Input: part model. Units: mm. Frame: model coordinates. A direction names the side the tool comes from. Coordinates: 2 decimals unless noted, no trailing zeros. Order: outer loops, then holes, each group sorted by start corner. A loop starts at its lowest first (then second) coordinate and runs counter-clockwise, first axis right, second up. Notation, with made-up numbers: M 17,55 L 70,55 A21 ccw 70,79 Z; hole C -36,77.25 d6. An arc over 180 degrees is marked long. Answer in a Markdown table with one row per item.
from build123d import *

# Parameters (mm, degrees)
SKETCH_1_W          = 830
SKETCH_1_H          = 82.91
EXTRUDE_2_DEPTH     = 20
SKETCH_4_W          = 830
SKETCH_4_H          = 10
CUT_EXTRUDE_3_DEPTH = 70
SKETCH_5_W          = 830
SKETCH_5_H          = 15
EXTRUDE_3_DEPTH     = 3.28
SKETCH_6_W          = 3.54
SKETCH_6_H          = 69.4
EXTRUDE_5_DEPTH     = 200.2
SKETCH_8_W          = 20
SKETCH_8_H          = 10.39973114
CUT_EXTRUDE_5_DEPTH = 1000.2
SKETCH_9_W          = 8.730890719
SKETCH_9_H          = 180.752173936
EXTRUDE_6_DEPTH     = 3.62
SKETCH_10_W         = 3.09
SKETCH_10_H         = 69.4
EXTRUDE_7_DEPTH     = 820
SKETCH_13_W         = 830
SKETCH_13_H         = 20
EXTRUDE_18_DEPTH    = 3.85


with BuildPart() as part:
    # 草图1 → 凸台-拉伸2 (new body)
    with BuildSketch(Plane.XY):
        with Locations((337.654216889, 6.096927721)):
            Rectangle(SKETCH_1_W, SKETCH_1_H)
    extrude(amount=EXTRUDE_2_DEPTH)

    # 草图4 → 切除-拉伸3 (cut)
    with BuildSketch(Plane(origin=(0, 47.551927721, 0), x_dir=(1, 0, 0), z_dir=(0, 1, 0))):
        with Locations((337.654216889, -15)):
            Rectangle(SKETCH_4_W, SKETCH_4_H)
    extrude(amount=-CUT_EXTRUDE_3_DEPTH, mode=Mode.SUBTRACT)

    # 草图5 → 凸台-拉伸3 (add)
    with BuildSketch(Plane(origin=(0, 47.551927721, 0), x_dir=(1, 0, 0), z_dir=(0, 1, 0))):
        with Locations((337.654216889, -7.5)):
            Rectangle(SKETCH_5_W, SKETCH_5_H)
    extrude(amount=EXTRUDE_3_DEPTH)

    # 草图6 → 凸台-拉伸5 (add)
    with BuildSketch(Plane(origin=(752.654216889, 50.831927721, 0), x_dir=(-1, 0, 0), z_dir=(0, 0, -1))):
        with Locations((1.77, -37.215224989)):
            Rectangle(SKETCH_6_W, SKETCH_6_H)
    extrude(amount=-EXTRUDE_5_DEPTH)

    # 草图8 → 切除-拉伸5 (cut)
    with BuildSketch(Plane.ZY.offset(77.345783111)):
        with Locations((10, -30.158206709)):
            Rectangle(SKETCH_8_W, SKETCH_8_H)
    extrude(amount=-CUT_EXTRUDE_5_DEPTH, mode=Mode.SUBTRACT)

    # 草图9 → 凸台-拉伸6 (add)
    with BuildSketch(Plane.XZ.offset(21.083297268)):
        with Locations((748.455599967, 110.153891103)):
            Rectangle(SKETCH_9_W, SKETCH_9_H)
    extrude(amount=EXTRUDE_6_DEPTH)

    # 草图10 → 凸台-拉伸7 (add)
    with BuildSketch(Plane.ZY.offset(-749.114216889)):
        with Locations((99.616509489, 13.616702732)):
            Rectangle(SKETCH_10_W, SKETCH_10_H)
    extrude(amount=EXTRUDE_7_DEPTH)

    # 草图13 → 凸台-拉伸18 (add)
    with BuildSketch(Plane(origin=(0, 48.316702732, 0), x_dir=(1, 0, 0), z_dir=(0, 1, 0))):
        with Locations((337.654216889, -108.539027645)):
            Rectangle(SKETCH_13_W, SKETCH_13_H)
    extrude(amount=EXTRUDE_18_DEPTH)


solid = part.part
1) Reachability of faces 4 (the face through (-77.346, 12, 3)), 5 (the face through (749.114, 13, 150)), 6 (the face through (332, 50.832, 7)) from +Z, -Z, +X, -X, +Y, -Y: full face, straight path, thin tool, end or side. Return the list, or none.
Resolved:
| item | result |
|---|---|
| face 4 | +Z, -Z, -X, +Y, -Y |
| face 5 | +Z, -X |
| face 6 | -Z, +X, -X, +Y |
2) Material intervals for probe 1 along Z at (x, y) = (318, 12.5); probe 2 along X at (y, z) = (29, 46), sorted ascending.
Resolved:
| item | result |
|---|---|
| probe 1 | z = 0 to 10, 98.07 to 101.16 |
| probe 2 | x = 749.11 to 752.65 |
3) Cut plane A-A, the plane x = 361. Output: boundary loops of the cut face in (y, z).
Resolved:
| item | result |
|---|---|
| outline | M -24.96,0 L 50.83,0 L 50.83,15 L 47.55,15 L 47.55,10 L -22.45,10 L -22.45,20 L -24.96,20 Z; M -21.08,98.07 L 48.32,98.07 L 48.32,98.54 L 52.17,98.54 L 52.17,118.54 L 48.32,118.54 L 48.32,101.16 L -21.08,101.16 Z |
4) Cut plane C-C, the plane z = 172.5. Output: boundary loops of the cut face in (x, y).
Resolved:
| item | result |
|---|---|
| outline | M 744.09,-24.7 L 752.82,-24.7 L 752.82,-21.08 L 752.65,-21.08 L 752.65,48.32 L 749.11,48.32 L 749.11,-21.08 L 744.09,-21.08 Z |
5) Mould query, pull axis Y, two halves, no side actions, for faces 1 (the face through (343, 13, 0)), 2 (the face through (332, 13, 10)), 3 (the face through (332, 52.167, 108)). Classes: +Y half, -Y half, draft (parallel to the pull), parting line (faces both ways), or undercut.
Resolved:
| item | result |
|---|---|
| face 1 | draft |
| face 2 | undercut |
| face 3 | +Y half |
6) Cut plane B-B, the plane y = 40. Output: boundary loops of the cut face in (x, z).
Resolved:
| item | result |
|---|---|
| outline | M -77.35,0 L 752.65,0 L 752.65,200.2 L 749.11,200.2 L 749.11,101.16 L -70.89,101.16 L -70.89,98.07 L 749.11,98.07 L 749.11,10 L -77.35,10 Z |
7) Contact query for flat-ended pins moving along their axis: pin 1 (1.6 mm diameter, centred on x = 141, y = 49, fed in from +Z); pin 2 (4 mm diameter, centred on x = 599.5, y = 37.5, fed in from +Z); pin 3 (11 mm diameter, centred on x = 349, z = 15.5, fed in from +Y). Output: stop coordinate, or through.
Resolved:
| item | result |
|---|---|
| pin 1 | stops at z = 118.54 |
| pin 2 | stops at z = 101.16 |
| pin 3 | stops at y = 50.83 |
